from build123d import *

# Parameters (mm, degrees)
SKETCH1_W           = 5.08
SKETCH1_H           = 5.08
BOSS_EXTRUDE1_DEPTH = 5.715
SKETCH2_W           = 65.16
SKETCH2_H           = 60.16
BOSS_EXTRUDE2_DEPTH = 5.08
FILLET1_R           = 5.08
SKETCH3_W           = 55
SKETCH3_H           = 50
BOSS_EXTRUDE3_DEPTH = 3.81
CUT_EXTRUDE1_DEPTH  = 3.81


with BuildPart() as part:
    # Sketch1 → Boss-Extrude1 (new body)
    with BuildSketch(Plane(origin=(0, 0, 0), x_dir=(1, 0, 0), z_dir=(0, 1, 0))):
        Polygon((-5.08, 0), (0, 0), (0, 50), (55, 50), (55, 55.08), (-5.08, 55.08), align=None)
        Polygon((55, 0), (0, 0), (0, -5.08), (60.08, -5.08), (60.08, 50), (55, 50), align=None)
        with Locations((-2.54, -2.54)):
            Rectangle(SKETCH1_W, SKETCH1_H)
        with Locations((57.54, 52.54)):
            Rectangle(SKETCH1_W, SKETCH1_H)
    extrude(amount=-BOSS_EXTRUDE1_DEPTH)

    # Sketch2 → Boss-Extrude2 (add)
    with BuildSketch(Plane(origin=(0, -5.715, 0), x_dir=(-1, 0, 0), z_dir=(0, -1, 0))):
        with Locations((-27.5, 25)):
            Rectangle(SKETCH2_W, SKETCH2_H)
    extrude(amount=BOSS_EXTRUDE2_DEPTH)

    # Fillet1
    fillet1_edges = [part.edges().sort_by_distance(p)[0] for p in [
        (-5.08, -5.3975, 5.08),
        (-5.08, -5.3975, -55.08),
        (60.08, -5.3975, -55.08),
        (60.08, -5.3975, 5.08),
        (-5.08, -10.795, -25),
        (27.5, -10.795, -55.08),
        (60.08, -10.795, -25),
        (27.5, -10.795, 5.08),
    ]]
    fillet(fillet1_edges, radius=FILLET1_R)

    # Sketch3 → Boss-Extrude3 (add)
    with BuildSketch(Plane(origin=(0, -5.715, 0), x_dir=(1, 0, 0), z_dir=(0, 1, 0))):
        with Locations((27.5, 25)):
            Rectangle(SKETCH3_W, SKETCH3_H)
    extrude(amount=BOSS_EXTRUDE3_DEPTH)

    # Sketch4 → Cut-Extrude1 (cut)
    with BuildSketch(Plane(origin=(0, -1.905, 0), x_dir=(1, 0, 0), z_dir=(0, 1, 0))):
        Polygon((27.5, 25), (52.25, 47.5), (2.75, 47.5), align=None)
        Polygon((52.9, 47.5), (52.25, 47.5), (27.5, 25), (52.25, 2.5), (52.9, 2.5), align=None)
        Polygon((52.25, 2.5), (27.5, 25), (2.75, 2.5), align=None)
        Polygon((2.75, 2.5), (27.5, 25), (2.75, 47.5), (2.1, 47.5), (2.1, 2.5), align=None)
    extrude(amount=-CUT_EXTRUDE1_DEPTH, mode=Mode.SUBTRACT)


solid = part.part
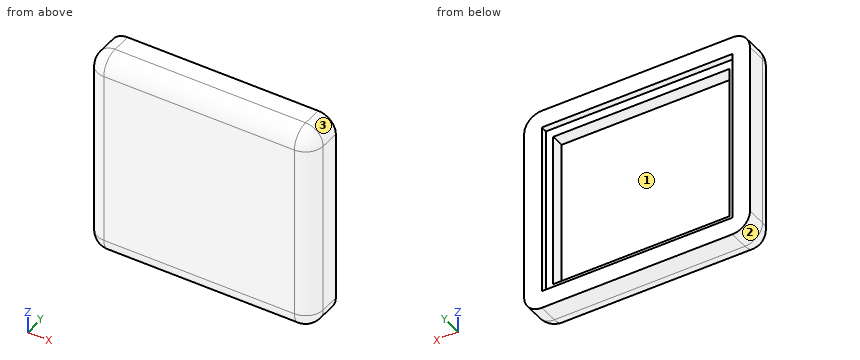
Geometry: final body of the model. Coordinates: model frame, mm. Face numbers are marked on the shaded views. Give positions to 0.01 mm unless a question says otherwise; leave off trailing zeros. Loops run counter-clockwise (first coordinate to the right, second up) from the corner with the lowest first, then second, coordinate; pieces in that order, holes last. Notation, with made-up numbers: (-33, 73) - (18, 73) arc R28 cw to (18, 105) - close; hole circle Ø8 at (-14.75, -23.75). An arc over 180 degrees is marked (long way). Answer as CSV lines item,"result". Start each with the question number.
1. Section A-A, the plane y = -2.75. Return loops of the section in (x, z), plus the area to 3 significant figures.
2. Section D-D, the plane y = -7. Return loops of the section in (x, z).
3. Section C-C, the plane x = 8. Return loops of the section in (y, z) (3 decimals).
4. Draft query along X for the marked faces 1, 2 and 3. Return one class per face: released by +X, released by -X, zero draft, split by the parting line, or undercut.
5. Pin query (flat end, axial travel): P1, Ø5, axis at x = 3.5, y = -6, coming from the +Z side; P2, Ø15, axis at x = 35, z = -31, coming from the +Y side (3 decimals); P3, Ø5, axis at x = 37, y = -9, coming from the +Z side. Return the tip coordinate at first contact, or that it passes through.
6. Ray query, L1, parallel to Z at x = 6, y = -3.5; L2, parallel to X at y = -0.25, z = -39.5; L3, parallel to X at y = -4, z = -25. Return the intervals inside material, ascending.
7. Section B-B, the plane z = -5.5. Return loops of the section in (x, y) (3 decimals).
Answers:
1,outline,"(-5.08, -50) arc R5.08 ccw to (0, -55.08) - (55, -55.08) arc R5.08 ccw to (60.08, -50) - (60.08, 0) arc R5.08 ccw to (55, 5.08) - (0, 5.08) arc R5.08 ccw to (-5.08, 0) - close; hole (2.1, -47.5) - (52.9, -47.5) - (52.9, -2.5) - (2.1, -2.5) - close"
1,area,"1,610 mm2"
2,outline,"(-4.91, -50) arc R4.91 ccw to (0, -54.91) - (55, -54.91) arc R4.91 ccw to (59.91, -50) - (59.91, 0) arc R4.91 ccw to (55, 4.91) - (0, 4.91) arc R4.91 ccw to (-4.91, 0) - close"
3,outline,"(-10.795, -50) arc R5.08 ccw to (-5.715, -55.08) - (0, -55.08) - (0, -50) - (-1.905, -50) - (-1.905, -47.5) - (-5.715, -47.5) - (-5.715, -2.5) - (-1.905, -2.5) - (-1.905, 0) - (0, 0) - (0, 5.08) - (-5.715, 5.08) arc R5.08 ccw to (-10.795, 0) - close"
4,face 1,"undercut"
4,face 2,"released by -X"
4,face 3,"released by +X"
5,P1,"stops at z = 5.08"
5,P2,"stops at y = -5.715"
5,P3,"stops at z = 5.02"
6,L1,"z = -55.08 to -47.5, -2.5 to 5.08"
6,L2,"x = -5.08 to 0, 55 to 60.08"
6,L3,"x = -5.08 to 2.1, 52.9 to 60.08"
7,outline,"(-5.08, -5.715) arc R5.08 ccw to (0, -10.795) - (55, -10.795) arc R5.08 ccw to (60.08, -5.715) - (60.08, 0) - (55, 0) - (55, -1.905) - (52.9, -1.905) - (52.9, -5.715) - (2.1, -5.715) - (2.1, -1.905) - (0, -1.905) - (0, 0) - (-5.08, 0) - close"
